```python
from build123d import *

# Parameters (mm, degrees)
SKETCH1_R           = 3.2639
SKETCH1_R_2         = 14.2875
SKETCH1_R_3         = 2.4892
BOSS_EXTRUDE1_DEPTH = 4.7625


with BuildPart() as part:
    # Sketch1 → Boss-Extrude1 (new body)
    with BuildSketch(Plane.XY):
        Polygon((0, 0), (76.2, 0), (76.2, 25.4), (50.8, 76.2), (25.4, 76.2), (0, 25.4), align=None)
        with Locations(Location((38.1, 12.7, 0), (0, 0, 180))):
            Circle(SKETCH1_R, mode=Mode.SUBTRACT)
        with Locations(Location((63.5, 12.7, 0), (0, 0, 180))):
            Circle(SKETCH1_R, mode=Mode.SUBTRACT)
        with Locations(Location((12.7, 12.7, 0), (0, 0, 180))):
            Circle(SKETCH1_R, mode=Mode.SUBTRACT)
        with Locations(Location((38.1, 50.8, 0), (0, 0, 180))):
            Circle(SKETCH1_R_2, mode=Mode.SUBTRACT)
        with Locations(Location((38.1, 31.75, 0), (0, 0, 180))):
            Circle(SKETCH1_R_3, mode=Mode.SUBTRACT)
    extrude(amount=BOSS_EXTRUDE1_DEPTH)


solid = part.part
```
Part model, mm, in its own coordinate system. Coordinates: 2 decimals unless noted, no trailing zeros. Loops run counter-clockwise (first coordinate to the right, second up) from the corner with the lowest first, then second, coordinate; pieces in that order, holes last. Notation, with made-up numbers: (29.5, -27) - (41.5, -27) arc R18 ccw to (41.5, 2) - close; hole circle Ø8 at (-6, 80). An arc over 180 degrees is marked (long way). Write item = value, one per line. Start each with the question number.
Item 1: Cut at C-C, the plane y = 53. Give the cut face in (x, z).
Item 2: Wall check: L1, parallel to X at y = 12.7, z = 3.55; L2, parallel to Y at x = 38.1, z = 2.1; L3, parallel to X at y = 11, z = 0.25. Give the ranges that are in metal, low to high. Write a range as from..to.
Item 3: Cut at A-A, the plane x = 38.1. Give the cut face in (y, z), and give its area (3 significant figures).
Item 4: Cut at D-D, the plane x = 47. Give the cut face in (y, z).
Item 5: Mould opens along X. For faces 1 (the cylindrical face through (13.125, 9.464, 2.348)), 2 (the flat face through (29, 30, 0)), 3 (the flat face through (76.2, 13, 2)), 4 (the flat face through (0, 13, 2)) say: released by +X, released by -X, zero draft, split by the parting line, or undercut.
Item 6: Flat gauge pins, fed straight in: pin 1 Ø2 at (y, z) = (45.5, 2.5) entering from +X; pin 2 Ø1.5 at (y, z) = (28, 1.5) entering from +X (3 decimals); pin 3 Ø10 at (x, y) = (46.5, 47.5) entering from -Z. Where does each tip first touch, or does it go through?
Item 7: Cut at B-B, the plane z = 3.5. State how many separate pieces and enclosed holes the cut face has, and give its area (3 significant figures).
The answers:
q1.outline = (13.8, 0) - (23.98, 0) - (23.98, 4.76) - (13.8, 4.76) - close; (52.22, 0) - (62.4, 0) - (62.4, 4.76) - (52.22, 4.76) - close
q2.L1 = 0..9.44, 15.96..34.84, 41.36..60.24, 66.76..76.2
q2.L2 = 0..9.44, 15.96..29.26, 34.24..36.51, 65.09..76.2
q2.L3 = 0..9.91, 15.49..35.31, 40.89..60.71, 66.29..76.2
q3.outline = (0, 0) - (9.44, 0) - (9.44, 4.76) - (0, 4.76) - close; (15.96, 0) - (29.26, 0) - (29.26, 4.76) - (15.96, 4.76) - close; (34.24, 0) - (36.51, 0) - (36.51, 4.76) - (34.24, 4.76) - close; (65.09, 0) - (76.2, 0) - (76.2, 4.76) - (65.09, 4.76) - close
q3.area = 172 mm2
q4.outline = (0, 0) - (39.62, 0) - (39.62, 4.76) - (0, 4.76) - close; (61.98, 0) - (76.2, 0) - (76.2, 4.76) - (61.98, 4.76) - close
q5.face_1 = undercut
q5.face_2 = zero draft
q5.face_3 = released by +X
q5.face_4 = released by -X
q6.pin_1 = 66.65
q6.pin_2 = 75.275
q6.pin_3 = through
q7.separate_pieces = 1
q7.enclosed_holes = 5
q7.area = 3,750 mm2
